```python
from build123d import *

# Parameters (mm, degrees)
SKETCH2_RX          = 22.5
SKETCH2_RY          = 7.5
SKETCH2_R           = 1.75
BOSS_EXTRUDE3_DEPTH = 3.5
SKETCH3_R           = 6
BOSS_EXTRUDE4_DEPTH = 10
CUT_EXTRUDE1_DEPTH  = 6.5


with BuildPart() as part:
    # Sketch2 → Boss-Extrude3 (new body)
    with BuildSketch(Plane(origin=(0, 0, 0), x_dir=(1, 0, 0), z_dir=(0, 1, 0))):
        with Locations((0, 0)):
            Ellipse(SKETCH2_RX, SKETCH2_RY)
        with Locations(Location((17.5, 0, 0), (0, 0, 270))):
            Circle(SKETCH2_R, mode=Mode.SUBTRACT)
        with Locations(Location((-17.5, 0, 0), (0, 0, 90))):
            Circle(SKETCH2_R, mode=Mode.SUBTRACT)
    extrude(amount=BOSS_EXTRUDE3_DEPTH)

    # Sketch3 → Boss-Extrude4 (add)
    with BuildSketch(Plane(origin=(0, 3.5, 0), x_dir=(1, 0, 0), z_dir=(0, 1, 0))):
        with Locations(Location((0, 0, 0), (0, 0, 270))):
            Circle(SKETCH3_R)
    extrude(amount=BOSS_EXTRUDE4_DEPTH)

    # Sketch4 → Cut-Extrude1 (cut)
    with BuildSketch(Plane(origin=(0, 13.5, 0), x_dir=(1, 0, 0), z_dir=(0, 1, 0))):
        Polygon((2.020725942, -3.5), (4.041451884, 0), (2.020725942, 3.5), (-2.020725942, 3.5), (-4.041451884, 0), (-2.020725942, -3.5), align=None)
    extrude(amount=-CUT_EXTRUDE1_DEPTH, mode=Mode.SUBTRACT)


solid = part.part
```
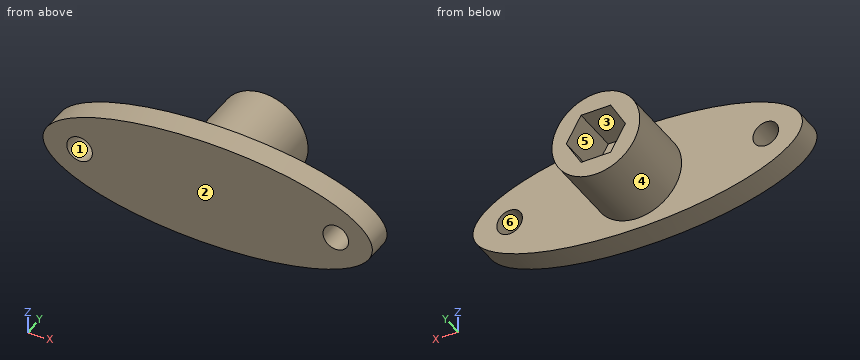
Could you check a few things on this model? Use its own coordinates, in mm. Face numbers are marked on the shaded views. A direction names the side the tool comes from. Round coordinates to 2 decimals unless told otherwise and drop trailing zeros. Loops run counter-clockwise (first coordinate to the right, second up) from the corner with the lowest first, then second, coordinate; pieces in that order, holes last. Notation, with made-up numbers: (63.25, -28) -> (70.25, -28) arc R11 ccw to (70.25, -13) -> close; hole circle Ø5 at (-19, 40). An arc over 180 degrees is marked (long way). Put each result on its own line as item: value.
Q1. Please list where these lines run through material, in increasing order: line 1 (X direction, y = 2.5, z = 0); line 2 (X direction, y = 1.5, z = -0.75); line 3 (Y direction, x = 1.5, z = -6). Write a range as from..to.
Checks:
line 1: -22.5..-19.25, -15.75..15.75, 19.25..22.5
line 2: -22.39..-19.08, -15.92..15.92, 19.08..22.39
line 3: 0..3.5
Q2. I want a section at B-B on y = 3. Give the number of separate pieces and of enclosed holes in the cut face, and give its area (3 significant figures).
Checks:
separate pieces: 1
enclosed holes: 2
area: 511 mm2
Q3. For pin 1 Ø3 at (x, y) = (-5, 11.5) entering from +Z; pin 2 Ø5.5 at (x, z) = (-17.5, 0) entering from +Y; pin 3 Ø1.2 at (x, y) = (0.5, 9) entering from +Z, each with a flat end and sliding along its axis, tell me the tip position at first contact or that it passes through.
Checks:
pin 1: z = 4.87
pin 2: y = 3.5
pin 3: z = 6
Q4. I want a section at A-A on y = 11.75. Write out the boundary of the cut face in (x, z).
Checks:
outline: circle Ø12 at (0, 0); hole (-4.04, 0) -> (-2.02, -3.5) -> (2.02, -3.5) -> (4.04, 0) -> (2.02, 3.5) -> (-2.02, 3.5) -> close
Q5. Which directions (+Z, -Z, +X, -X, +Y, -Y) give clear straight access to the entire face, cutting with the end or side of a thin tool? Please do the marked faces 5 and 6.
Checks:
face 5: +Y
face 6: +Y, -Y
Q6. Thinking about a two-plate mould opening in X: for the marked faces 1, 2, 3 and 4, which applies, pulls with the +X half, pulls with the -X half, needs draft (parallel to the pull), parting line crosses it, or undercut?
Checks:
face 1: undercut
face 2: needs draft
face 3: undercut
face 4: parting line crosses it
